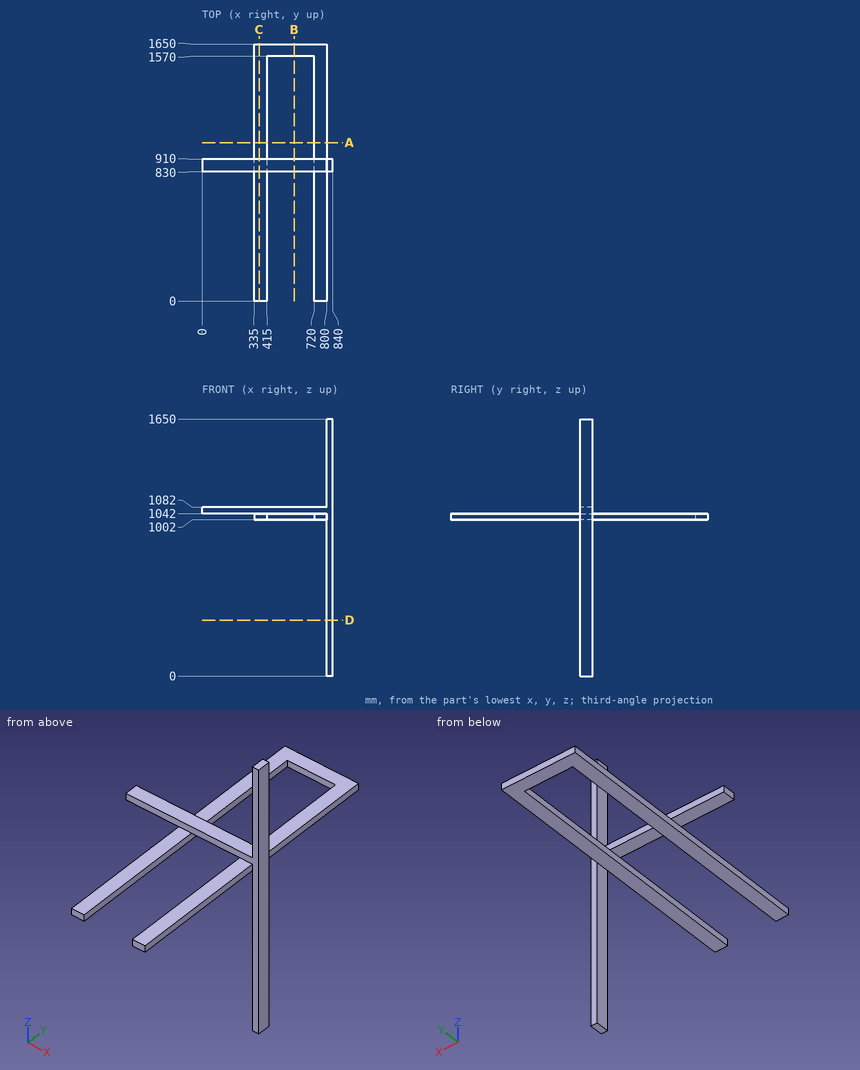
The figure shows three views and two pictorial views of one solid part (mm, origin at its lowest corner). Answer the questions. Give positions to 0.01 mm unless a question says otherwise; leave off trailing zeros. Write each loop counter-clockwise with the first axis right and the second up, starting at its lowest first coordinate (ties: lowest second). Pieces come first, ordered by that corner, then holes.
Q1. Straight lines are drawn through the part: L1, parallel to Z at x = 798, y = 516; L2, parallel to Y at x = 549, z = 1020.5; L3, parallel to Z at x = 177.5, y = 905. For each, find the intervals that lie inside material, in ascending order.
Answer:
L1: z = 1002 to 1042
L2: y = 1570 to 1650
L3: z = 1042 to 1082
Q2. The part is cut by section A-A on y = 1017. Give the vertices of the cut face in (x, z).
Answer:
outline: (335, 1002) - (415, 1002) - (415, 1042) - (335, 1042) - close; (720, 1002) - (800, 1002) - (800, 1042) - (720, 1042) - close
Q3. The part is cut by section B-B on x = 591. Give the vertices of the cut face in (y, z), and give its area (3 significant figures).
Answer:
outline: (830, 1042) - (910, 1042) - (910, 1082) - (830, 1082) - close; (1570, 1002) - (1650, 1002) - (1650, 1042) - (1570, 1042) - close
area: 6,400 mm2
Q4. The part is cut by section C-C on x = 367. Give the vertices of the cut face in (y, z), and give its area (3 significant figures).
Answer:
outline: (0, 1002) - (1650, 1002) - (1650, 1042) - (910, 1042) - (910, 1082) - (830, 1082) - (830, 1042) - (0, 1042) - close
area: 69,200 mm2
Q5. Given pin 1 (24 mm diameter, centred on x = 368, y = 217, fed in from +Z); pin 2 (20 mm diameter, centred on y = 1109.5, z = 1026, fed in from +X); pin 3 (24 mm diameter, centred on y = 878.5, z = 1421.5, fed in from -X), each flat-ended and moving along its own axis, determine where each tip first touches the part or whether it passes through.
Answer:
pin 1: stops at z = 1042
pin 2: stops at x = 800
pin 3: stops at x = 800
Q6. The part is cut by section D-D on z = 358. Give the vertices of the cut face in (x, y).
Answer:
outline: (800, 830) - (840, 830) - (840, 910) - (800, 910) - close
